Check sheet for the modelled part. Datum: model origin and axes. Units: mm. A direction names the side the tool comes from. Give positions to 0.01 mm unless a question says otherwise; leave off trailing zeros. Loops run counter-clockwise (first coordinate to the right, second up) from the corner with the lowest first, then second, coordinate; pieces in that order, holes last. Notation, with made-up numbers: (-13.75, -9) - (-4.75, -9) arc R22 cw to (-4.75, 16) - close; hole circle Ø1 at (69.5, 25). An arc over 180 degrees is marked (long way). Use one line per item in the form item = value.
from build123d import *

# Parameters (mm, degrees)
BASE_EXTRUDE_DEPTH = 12.7


with BuildPart() as part:
    # Sketch1 → Base-Extrude (new, symmetric)
    with BuildSketch(Plane.XY):
        with BuildLine():
            Line((-20.6375, 29.1719), (-20.6375, -25.3238))
            ThreePointArc((-20.6375, -25.3238), (-19.848914298, -27.227614298), (-17.9451, -28.0162))
            Line((-17.9451, -28.0162), (17.9451, -28.0162))
            ThreePointArc((17.9451, -28.0162), (19.848914298, -27.227614298), (20.6375, -25.3238))
            Line((20.6375, -25.3238), (20.6375, 29.1719))
            ThreePointArc((20.6375, 29.1719), (15.875, 33.9344), (11.1125, 29.1719))
            Line((11.1125, 29.1719), (11.1125, 28.13685))
            ThreePointArc((11.1125, 28.13685), (12.4587, 26.79065), (13.8049, 28.13685))
            Line((13.8049, 28.13685), (13.8049, 29.1719))
            ThreePointArc((13.8049, 29.1719), (15.875, 31.242), (17.9451, 29.1719))
            Line((17.9451, 29.1719), (17.9451, -25.3238))
            Line((17.9451, -25.3238), (-17.9451, -25.3238))
            Line((-17.9451, -25.3238), (-17.9451, 29.1719))
            ThreePointArc((-17.9451, 29.1719), (-15.875, 31.242), (-13.8049, 29.1719))
            Line((-13.8049, 29.1719), (-13.8049, 28.13685))
            ThreePointArc((-13.8049, 28.13685), (-12.4587, 26.79065), (-11.1125, 28.13685))
            Line((-11.1125, 28.13685), (-11.1125, 29.1719))
            ThreePointArc((-11.1125, 29.1719), (-15.875, 33.9344), (-20.6375, 29.1719))
        make_face()
    extrude(amount=BASE_EXTRUDE_DEPTH, both=True)


solid = part.part
Item 1: Section check D-D on x = 5. Record the boundary of the cut face in (y, z), then the cut area to 3 significant figures.
Answer block:
outline = (-28.02, -12.7) - (-25.32, -12.7) - (-25.32, 12.7) - (-28.02, 12.7) - close
area = 68.4 mm2
Item 2: Section check B-B on z = -0.5. Record the boundary of the cut face in (x, y) (1 decimal).
Answer block:
outline = (-20.6, -25.3) arc R2.7 ccw to (-17.9, -28) - (17.9, -28) arc R2.7 ccw to (20.6, -25.3) - (20.6, 29.2) arc R4.8 ccw to (11.1, 29.2) - (11.1, 28.1) arc R1.3 ccw to (13.8, 28.1) - (13.8, 29.2) arc R2.1 cw to (17.9, 29.2) - (17.9, -25.3) - (-17.9, -25.3) - (-17.9, 29.2) arc R2.1 cw to (-13.8, 29.2) - (-13.8, 28.1) arc R1.3 ccw to (-11.1, 28.1) - (-11.1, 29.2) arc R4.8 ccw to (-20.6, 29.2) - close
Item 3: Section check C-C on x = 12.5. Record the boundary of the cut face in (y, z).
Answer block:
outline = (-28.02, -12.7) - (-25.32, -12.7) - (-25.32, 12.7) - (-28.02, 12.7) - close; (26.79, -12.7) - (32.53, -12.7) - (32.53, 12.7) - (26.79, 12.7) - close
Item 4: Access from +Z, -Z, +X, -X, +Y, -Y to the whole of each face (thin tool, end or side, straight path). Record for faces 1 (the face through (-18.4, 0.8, -12.7)), 2 (the face through (0, -25.324, 0)).
Answer block:
face_1 = -Z, +X, -X, +Y, -Y
face_2 = +Z, -Z
Item 5: Mould release check, pull along Y, two halves, no side actions. Record for faces 3 (the face through (-19.87, -27.207, 0.178)), 4 (the face through (-20.638, 2, 0)), 5 (the face through (-17.945, 2, 0)): released by +Y, released by -Y, zero draft, split by the parting line, or undercut.
Answer block:
face_3 = released by -Y
face_4 = zero draft
face_5 = undercut
Item 6: Section check A-A on y = 23.5. Record the boundary of the cut face in (x, z), then the cut area to 3 significant figures.
Answer block:
outline = (-20.64, -12.7) - (-17.95, -12.7) - (-17.95, 12.7) - (-20.64, 12.7) - close; (17.95, -12.7) - (20.64, -12.7) - (20.64, 12.7) - (17.95, 12.7) - close
area = 137 mm2
Item 7: Gauge pin test, flat end, axial feed: P1, Ø7.5, axis at x = -5.5, z = -3, coming from the +Y side. Record the tip position at first contact, or that the pin passes through.
Answer block:
P1 = -25.32
Item 8: Thickness scan on L1, parallel to X at y = -21, z = -10.75; L2, parallel to Y at x = 16, z = -11; L3, parallel to Y at x = -11, z = -0.25. Record the ranges inside material, lowest first.
Answer block:
L1 = -20.64 to -17.95, 17.95 to 20.64
L2 = -28.02 to -25.32, 31.24 to 33.93
L3 = -28.02 to -25.32
